Geometry: see drawing. Coordinates: mm, zero at the bounding-box minimum. Give positions to 0.01 mm unless a question says otherwise; leave off trailing zeros. Loops run counter-clockwise (first coordinate to the right, second up) from the corner with the lowest first, then second, coordinate; pieces in that order, holes last. Notation, with made-up numbers: (-21.5, 76.5) -> (27.5, 76.5) arc R16 ccw to (27.5, 94.5) -> close; hole circle Ø7 at (7.5, 64). An arc over 180 degrees is marked (long way). Use CSV: the item, a comma, the result in double quotes.
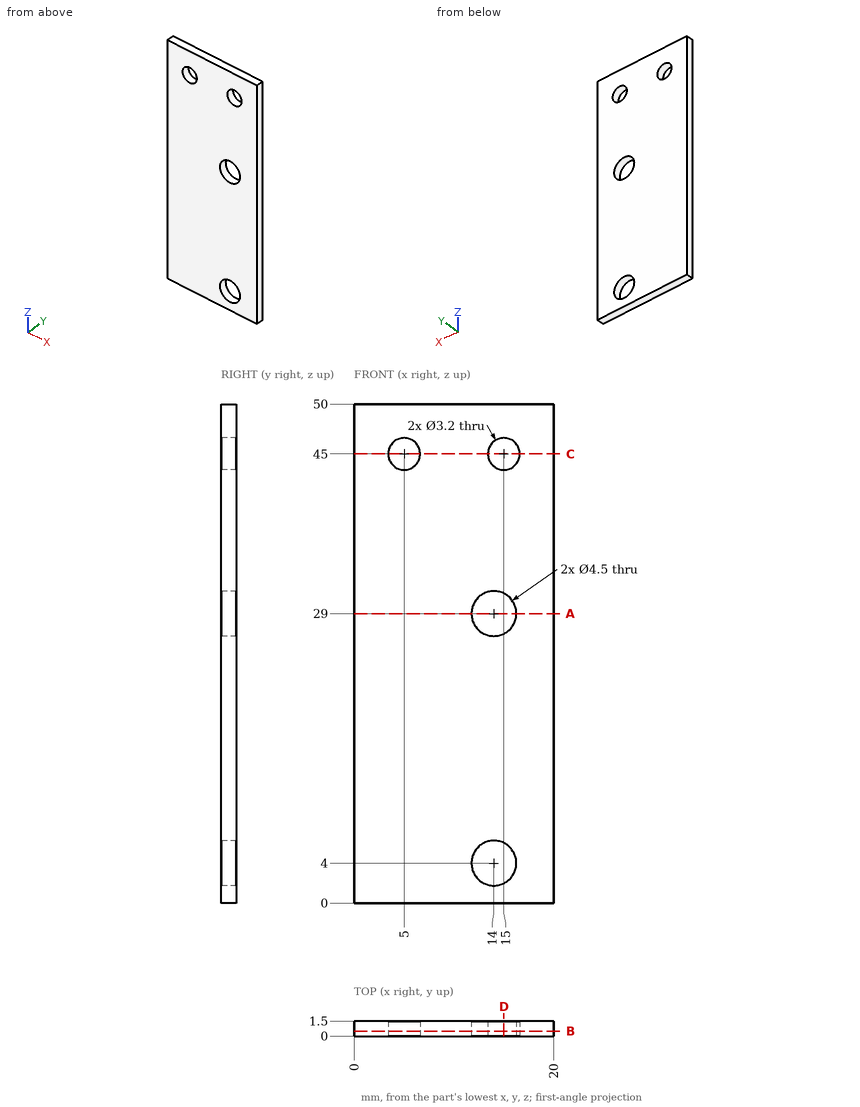
1) Section query A-A (z = 29). Return loops of the section in (x, y).
From the geometry:
outline,"(0, 0) -> (11.75, 0) -> (11.75, 1.5) -> (0, 1.5) -> close; (16.25, 0) -> (20, 0) -> (20, 1.5) -> (16.25, 1.5) -> close"
2) Section query B-B (y = 0.5). Return loops of the section in (x, z), then the cut area to 3 significant figures.
From the geometry:
outline,"(0, 0) -> (20, 0) -> (20, 50) -> (0, 50) -> close; hole circle Ø3.2 at (5, 45); hole circle Ø4.5 at (14, 4); hole circle Ø4.5 at (14, 29); hole circle Ø3.2 at (15, 45)"
area,"952 mm^2"
3) Section query C-C (z = 45). Return loops of the section in (x, y), then the cut area to 3 significant figures.
From the geometry:
outline,"(0, 0) -> (3.4, 0) -> (3.4, 1.5) -> (0, 1.5) -> close; (6.6, 0) -> (13.4, 0) -> (13.4, 1.5) -> (6.6, 1.5) -> close; (16.6, 0) -> (20, 0) -> (20, 1.5) -> (16.6, 1.5) -> close"
area,"20.4 mm^2"
4) Ray query, line 1 (X direction, y = 1.25, z = 45); line 2 (Z direction, x = 15, y = 0.65); line 3 (Z direction, x = 14, y = 1.25). Return the intervals inside material, ascending.
From the geometry:
line 1,"x = 0 to 3.4, 6.6 to 13.4, 16.6 to 20"
line 2,"z = 0 to 1.98, 6.02 to 26.98, 31.02 to 43.4, 46.6 to 50"
line 3,"z = 0 to 1.75, 6.25 to 26.75, 31.25 to 43.75, 46.25 to 50"
5) Section query D-D (x = 15). Return loops of the section in (y, z).
From the geometry:
outline,"(0, 0) -> (1.5, 0) -> (1.5, 1.98) -> (0, 1.98) -> close; (0, 6.02) -> (1.5, 6.02) -> (1.5, 26.98) -> (0, 26.98) -> close; (0, 31.02) -> (1.5, 31.02) -> (1.5, 43.4) -> (0, 43.4) -> close; (0, 46.6) -> (1.5, 46.6) -> (1.5, 50) -> (0, 50) -> close"
